For this review, take the finished solid that the model builds, in its own axes (mm). A direction names the side the tool comes from. Coordinates: 2 decimals unless noted, no trailing zeros. Write each loop counter-clockwise with the first axis right and the second up, starting at its lowest first coordinate (ties: lowest second). Pieces come first, ordered by that corner, then holes. Notation, with made-up numbers: (-3.75, 24.5) - (25.25, 24.5) arc R16 ccw to (25.25, 42.5) - close; hole circle Ø10 at (-29, 38.5). An arc over 180 degrees is marked (long way). Use one line per item in the form item = value. Start each with the question number.
1) We need section A-A (y = 2.25). Give the boundary of the cut face in (x, z).
2) For L1, parallel to Z at x = -153.5, y = -1.25; L2, parallel to X at y = -1.5, z = 103; L3, parallel to Y at x = -179, z = 67.5, list the stretches that pass through material, from the lowest coordinate up. Write a range as from..to.
3) Insertion check: P1, Ø1.2, axis at x = 81, y = -2, coming from the +Z side; P2, Ø4, axis at y = -0.5, z = 90, coming from the +X side; P3, Ø0.6, axis at y = 1, z = 163.5, coming from the -X side; P4, Ø2, axis at y = -5, z = -42, coming from the -X side. Each pin has a flat end and moves straight along its axis. Give the tip position at first contact, or say it passes through.
4) Tool access review of faces 1 (the cylindrical face through (-222.79, -1.23, 56.55)), 2 (the flat face through (235, -1, 162.727)): name each direction out of +Z, -Z, +X, -X, +Y, -Y from which nothing blocks a thin tool from reaching the whole face with its end or side.
5) We need section B-B (z = 121). Count the separate pieces of the cut face and the enclosed holes in it, plus the area to 3 significant figures.
6) Mouldability with a two-part tool opening along X and no side actions: class faces 3 (the cylindrical face through (-162.38, -1.23, 132.48)), 4 (the flat face through (-128, -2.5, 105)) as pulls with the +X half, pulls with the -X half, needs draft (parallel to the pull), parting line crosses it, or undercut.
```python
from build123d import *

# Parameters (mm, degrees)
F1_DEPTH = 2.5
F3_D     = 70
F4_D     = 35
F5_W     = 5
F5_H     = 2.5
F6_DEPTH = 2
F7_DEPTH = 0.1


with BuildPart() as f1:
    # F0 (on Front) → F1 (new body)
    with BuildSketch(Plane.XZ):
        with BuildLine():
            Line((234.3109268695, 164.7265180945), (-265.6890731305, 164.7265180945))
            Line((-265.6890731305, 164.7265180945), (-265.6890731305, -85.2734819055))
            Line((-265.6890731305, -85.2734819055), (-263.6890731305, -85.2734819055))
            add(Edge.make_bspline(
                [(234.3109268695, 162.7265180945), (-263.6890731305, 162.7265180945), (-263.6890731305, -85.2734819055)],
                knots=[4.7123889804, 4.7123889804, 4.7123889804, 6.2831853072, 6.2831853072, 6.2831853072], degree=2, weights=[1, 0.7071067812, 1]))
            Line((234.3109268695, 162.7265180945), (234.3109268695, 164.7265180945))
        make_face()
    extrude(amount=F1_DEPTH)

    # F3 (through all)
    with Locations(Plane.XZ.offset(2.5)):
        with Locations((-210.6890731305, 109.7265180945)):
            Hole(F3_D / 2)

    # F4 (through all)
    with Locations(Plane.XZ.offset(2.5)):
        with Locations((-145.6890731305, 127.2265180945), (-235.6890731305, 44.7265180945)):
            Hole(F4_D / 2)

    # F5 (on face) → F6 (join)
    with BuildSketch(Plane.XY.offset(164.7265180945)):
        Polygon((239.3109268695, -6.25), (239.3109268695, 3.75), (229.3109268695, 3.75), (229.3109268695, 0), (234.3109268695, 0), (234.3109268695, -2.5), (229.3109268695, -2.5), (229.3109268695, -6.25), align=None)
        with Locations((231.8109268695, -1.25)):
            Rectangle(F5_W, F5_H)
    extrude(amount=-F6_DEPTH)

    # F5 (on face) → F7 (join)
    with BuildSketch(Plane.XY.offset(164.7265180945)):
        Polygon((239.3109268695, -6.25), (239.3109268695, 3.75), (229.3109268695, 3.75), (229.3109268695, 0), (234.3109268695, 0), (234.3109268695, -2.5), (229.3109268695, -2.5), (229.3109268695, -6.25), align=None)
        with Locations((231.8109268695, -1.25)):
            Rectangle(F5_W, F5_H)
    extrude(amount=F7_DEPTH)


solid = f1.part
```
Determined:
q1.outline = (229.31, 162.73) - (239.31, 162.73) - (239.31, 164.83) - (229.31, 164.83) - close
q2.L1 = 70.31..111.57, 142.89..164.73
q2.L2 = -265.69..-245.04, -176.34..-89.84
q2.L3 = -2.5..0
q3.P1 = 164.73
q3.P2 = -113.95
q3.P3 = 229.31
q3.P4 = through
q4.face_1 = +Y, -Y
q4.face_2 = -Z, +X, +Y, -Y
q5.separate_pieces = 3
q5.enclosed_holes = 0
q5.area = 311 mm²
q6.face_3 = undercut
q6.face_4 = needs draft
